The listing builds one solid part. Answer for the finished solid, in the listing's coordinates (mm). A direction names the side the tool comes from. Give positions to 0.01 mm unless a question says otherwise; leave off trailing zeros. Write each loop counter-clockwise with the first axis right and the second up, starting at its lowest first coordinate (ties: lowest second). Pieces come first, ordered by that corner, then holes. Notation, with made-up numbers: (40, 52.5) -> (47, 52.5) arc R18 cw to (47, 56.5) -> close; hole circle Ø5 at (-12, 80.5). An arc over 180 degrees is marked (long way). Write each question's results on one line, items separated by ' | '. Start each with the question number.
from build123d import *

# Parameters (mm, degrees)
F1_DEPTH = 25.4


with BuildPart() as f1:
    # F0 (on Front) → F1 (new body)
    with BuildSketch(Plane.XZ):
        with BuildLine():
            Line((40.7043881714, -23.8888029385), (40.7043881714, 25.317851454))
            Line((40.7043881714, 25.317851454), (9.4020965094, 5.8480398177))
            ThreePointArc((9.4020965094, 5.8480398177), (10.6466699917, 3.0409548779), (11.0724427513, 0))
            ThreePointArc((11.0724427513, 0), (10.6848861314, -2.9038245196), (9.5493467137, -5.6043702432))
            Line((9.5493467137, -5.6043702432), (40.7043881714, -23.8888029385))
        make_face()
        with BuildLine():
            ThreePointArc((11.0724427513, 0), (10.6466699917, 3.0409548779), (9.4020965094, 5.8480398177))
            Line((9.4020965094, 5.8480398177), (0, 0))
            Line((0, 0), (9.5493467137, -5.6043702432))
            ThreePointArc((9.5493467137, -5.6043702432), (10.6848861314, -2.9038245196), (11.0724427513, 0))
        make_face()
        with BuildLine():
            Line((0, 0), (9.4020965094, 5.8480398177))
            ThreePointArc((9.4020965094, 5.8480398177), (0.6010385922, 11.0561178128), (-8.7127334808, 6.8328078982))
            Line((-8.7127334808, 6.8328078982), (0, 0))
        make_face()
        with BuildLine():
            ThreePointArc((-8.9241617805, -6.5542600647), (0.5685830796, -11.0578344065), (9.5493467137, -5.6043702432))
            Line((9.5493467137, -5.6043702432), (0, 0))
            Line((0, 0), (-8.9241617805, -6.5542600647))
        make_face()
        with BuildLine():
            Line((-8.9241617805, -6.5542600647), (0, 0))
            Line((0, 0), (-8.7127334808, 6.8328078982))
            ThreePointArc((-8.7127334808, 6.8328078982), (-11.0710620889, 0.1748505229), (-8.9241617805, -6.5542600647))
        make_face()
        with BuildLine():
            ThreePointArc((-8.9241617805, -6.5542600647), (-11.0710620889, 0.1748505229), (-8.7127334808, 6.8328078982))
            Line((-8.7127334808, 6.8328078982), (-33.7105058134, 26.4368709177))
            Line((-33.7105058134, 26.4368709177), (-33.7105058134, -24.7583389282))
            Line((-33.7105058134, -24.7583389282), (-8.9241617805, -6.5542600647))
        make_face()
    extrude(amount=F1_DEPTH)


solid = f1.part
1. A tool of negligible diameter and unlimited length cuts with its end or side. For faces 4 (the flat face through (3, 0, 1)), 5 (the flat face through (-21.491, -12.522, -15.784)), 6 (the flat face through (25.27, -12.52, 15.72)), from which of +Z, -Z, +X, -X, +Y, -Y can it reach the whole face along a straight path? Write none if from no direction.
2. The mould has two halves that part along X. Classify faces 1 (the flat face through (-33.711, -13, 1)), 2 (the flat face through (40.704, -13, 0)), 3 (the flat face through (-21.04, -12.52, 16.5)): pulls with the +X half, pulls with the -X half, needs draft (parallel to the pull), parting line crosses it, or undercut.
3. Section A-A (z = 17.5) is taken. Write down the section's boundary in (x, y), then the cut area to 3 significant figures.
4. Each of these flat-tipped pins is pushed along its axis until it touches: pin 1 Ø1.5 at (x, z) = (10, -3.5) entering from +Y; pin 2 Ø5 at (x, y) = (17, -8) entering from +Z; pin 3 Ø2 at (x, y) = (-9, -16.5) entering from +Z. Where does it stop, or does it pass through?
5. Consider probe 1 along X at (y, z) = (-2.25, -7); probe 2 along X at (y, z) = (-19, 9.5); probe 3 along X at (y, z) = (-2.5, -15). Determine where each line is inside the solid, lowest interval first. Write a range as [from, to].
6. Section D-D (x = -15.5) is taken. Write down the section's boundary in (y, z).
7. Section C-C (z = -9.5) is taken. Write down the section's boundary in (x, y), then the cut area to 3 significant figures.
8. Section B-B (y = -22) is taken. Write down the section's boundary in (x, z), then the cut area to 3 significant figures.
Results:
1) face 4: +Z, -Z, +X, -X, +Y | face 5: -Z, +Y, -Y | face 6: +Z, +Y, -Y
2) face 1: pulls with the -X half | face 2: pulls with the +X half | face 3: undercut
3) outline: (-33.71, -25.4) -> (-22.31, -25.4) -> (-22.31, 0) -> (-33.71, 0) -> close; (28.14, -25.4) -> (40.7, -25.4) -> (40.7, 0) -> (28.14, 0) -> close | area: 609 mm²
4) pin 1: stops at y = 0 | pin 2: stops at z = 12.13 | pin 3: stops at z = 7.84
5) probe 1: x = [-33.71, -9.53], [-8.58, 8.58], [11.93, 40.7] | probe 2: x = [-33.71, -12.11], [-5.69, 5.69], [15.27, 40.7] | probe 3: x = [-33.71, -20.42], [25.56, 40.7]
6) outline: (-25.4, -11.38) -> (0, -11.38) -> (0, 12.16) -> (-25.4, 12.16) -> close
7) outline: (-33.71, -25.4) -> (-12.94, -25.4) -> (-12.94, 0) -> (-33.71, 0) -> close; (-5.69, -25.4) -> (5.69, -25.4) -> (5.69, 0) -> (-5.69, 0) -> close; (16.19, -25.4) -> (40.7, -25.4) -> (40.7, 0) -> (16.19, 0) -> close | area: 1,440 mm²
8) outline: (-33.71, -24.76) -> (-8.92, -6.55) arc R11.07 ccw to (9.55, -5.6) -> (40.7, -23.89) -> (40.7, 25.32) -> (9.4, 5.85) arc R11.07 ccw to (-8.71, 6.83) -> (-33.71, 26.44) -> close | area: 2,100 mm²
